Autodesk Inventor part; units mm, degrees
ref_plane "YZ Plane" through (0, 0, 0) normal (1, 0, 0) x (0, 1, 0)
ref_plane "XZ Plane" through (0, 0, 0) normal (0, 1, 0) x (-1, 0, 0)
ref_plane "XY Plane" through (0, 0, 0) normal (0, 0, 1) x (1, 0, 0)
sketch "Boceto1" plane through (0, 0, 0) normal (0, 0, 1) x (1, 0, 0)
  line L0 (250, 0) -> (250, 1160)
  line L1 (0, 1160) -> (0, 0)
  line L2 (230, 20) -> (230, 0)
  line L3 (20, 20) -> (20, 0)
  line L4 (230, 0) -> (230, 140)
  line L5 (230, 140) -> (20, 140)
  line L6 (20, 152.5) -> (230, 152.5)
  line L7 (230, 152.5) -> (230, 457.5)
  line L8 (230, 457.5) -> (20, 457.5)
  line L9 (20, 457.5) -> (20, 470)
  line L10 (20, 470) -> (230, 470)
  line L11 (230, 470) -> (230, 457.5)
  line L12 (230, 470) -> (230, 775)
  line L13 (230, 775) -> (20, 775)
  line L14 (20, 775) -> (20, 787.5)
  line L15 (20, 787.5) -> (230, 787.5)
  line L16 (230, 787.5) -> (230, 775)
  line L17 (230, 787.5) -> (230, 1147.5)
  line L18 (230, 1147.5) -> (20, 1147.5)
  line L19 (20, 1160) -> (230, 1160)
  line L20 (230, 1160) -> (230, 1147.5)
  line L21 (0, 0) -> (20, 0)
  line L22 (230, 0) -> (250, 0)
  line L23 (20, 20) -> (20, 140)
  line L24 (230, 140) -> (230, 20)
  line L25 (20, 152.5) -> (20, 457.5)
  line L26 (230, 1147.5) -> (230, 470)
  line L27 (230, 457.5) -> (230, 152.5)
  line L28 (20, 470) -> (20, 775)
  line L29 (20, 787.5) -> (20, 1147.5)
  line L30 (0, 0) -> (529.2462, 0) construction
  line L31 (20, 1160) -> (0, 1160)
  line L32 (230, 1160) -> (250, 1160)
  line L33 (230, 1147.5) -> (250, 1147.5)
  dimension "d5" = 140
  dimension "d6" = 12.5
  dimension "d7" = 305
  dimension "d8" = 12.5
  dimension "d9" = 305
  dimension "d10" = 12.5
  dimension "d11" = 360
  dimension "d13" = 12.5
  dimension "d28" = 1160
  dimension "d29" = 250
  dimension "d30" = 210
  dimension "d31" = 20
extrude "Extrusión1" add sketch "Boceto1" along normal blind 600 contours L22 L2 L4 L5 L23 L3 L21 L1 L31 L19 L20 L33 L0 | L33 L20 L32 L0 | L16 L13 L14 L15 | L11 L8 L9 L10
sketch "Boceto2" plane through (250, 0, 0) normal (1, 0, 0) x (0, 0, -1)
  line L0 (0, 457.5) -> (0, 152.5)
  line L1 (0, 152.5) -> (0, 457.5)
  line L2 (0, 0) -> (-600, 0)
  line L3 (0, 0) -> (-600, 0)
  line L4 (0, 0) -> (-600, 0)
  line L5 (0, 0) -> (-600, 0)
  line L6 (-600, 140) -> (-600, 0)
  line L7 (0, 140) -> (0, 0)
  line L8 (0, 0) -> (-600, 0)
  line L9 (-600, 140) -> (-600, 0)
  line L10 (0, 140) -> (-600, 140)
  line L11 (0, 0) -> (-600, 0)
  line L12 (0, 0) -> (-600, 0)
  line L13 (0, 140) -> (-600, 140)
  line L14 (0, 0) -> (0, 140)
  line L15 (0, 140) -> (-600, 140)
  line L16 (-600, 0) -> (-600, 140)
  line L17 (0, 0) -> (-600, 0)
  line L18 (0, 140) -> (-600, 140)
  line L19 (0, 140) -> (-600, 140)
  line L20 (0, 152.5) -> (-600, 152.5)
  line L21 (-600, 457.5) -> (-600, 152.5)
  line L22 (0, 457.5) -> (0, 152.5)
  line L23 (0, 152.5) -> (-600, 152.5)
  line L24 (-600, 457.5) -> (-600, 152.5)
  line L25 (0, 457.5) -> (-600, 457.5)
  line L26 (-600, 152.5) -> (-600, 457.5)
  line L27 (0, 152.5) -> (0, 457.5)
  line L28 (0, 457.5) -> (-600, 457.5)
  line L29 (-600, 152.5) -> (-600, 457.5)
  line L30 (0, 152.5) -> (-600, 152.5)
  line L31 (0, 0) -> (0, 1160)
  line L32 (0, 1160) -> (0, 0)
  line L33 (0, 140) -> (0, 0)
  line L34 (0, 0) -> (0, 140)
  line L35 (0, 1160) -> (0, 0)
  line L36 (0, 0) -> (0, 1160)
  line L37 (0, 470) -> (0, 775)
  line L38 (0, 775) -> (0, 470)
  line L39 (0, 152.5) -> (0, 457.5)
  line L40 (0, 457.5) -> (0, 152.5)
  line L41 (-600, 0) -> (-600, 1160)
  line L42 (0, 0) -> (0, 1160)
  line L43 (-600, 0) -> (-600, 1160)
  line L44 (0, 0) -> (-600, 0)
  line L45 (-600, 1160) -> (-600, 0)
  line L46 (0, 1160) -> (0, 0)
  line L47 (0, 0) -> (-600, 0)
  line L48 (-600, 1160) -> (-600, 0)
  line L49 (-600, 140) -> (-600, 0)
  line L50 (-600, 0) -> (-600, 1160)
  line L51 (-600, 1160) -> (-600, 0)
  line L52 (-600, 0) -> (-600, 140)
  line L53 (-600, 470) -> (-600, 775)
  line L54 (-600, 775) -> (-600, 470)
  line L55 (-600, 457.5) -> (-600, 152.5)
  line L56 (-600, 152.5) -> (-600, 457.5)
  line L57 (0, 1600) -> (-600, 1600)
  line L58 (0, 152.5) -> (-600, 152.5)
  line L59 (0, 152.5) -> (-600, 152.5)
  line L60 (0, 152.5) -> (-600, 152.5)
  line L61 (0, 0) -> (-600, 0)
  line L62 (0, 140) -> (-600, 140)
  line L63 (0, 140) -> (0, 0)
  line L64 (-600, 0) -> (-600, 140)
  line L65 (0, 0) -> (-600, 0)
  line L66 (0, 0) -> (0, 140)
  line L67 (0, 1160) -> (-600, 1160)
  line L68 (0, 1160) -> (-600, 1160)
  line L69 (0, 1160) -> (0, 1147.5)
  line L70 (0, 1580) -> (-600, 1580)
  line L71 (0, 1580) -> (-600, 1580)
  line L72 (0, 1580) -> (0, 1160)
  line L73 (-600, 1160) -> (-600, 1147.5)
  line L74 (-600, 470) -> (-600, 775)
  line L75 (0, 457.5) -> (-600, 457.5)
  line L76 (0, 457.5) -> (-600, 457.5)
  line L77 (0, 457.5) -> (-600, 457.5)
  line L78 (0, 457.5) -> (-600, 457.5)
  line L79 (0, 470) -> (-600, 470)
  line L80 (0, 470) -> (-600, 470)
  line L81 (0, 470) -> (-600, 470)
  line L82 (-600, 775) -> (-600, 470)
  line L83 (0, 775) -> (0, 470)
  line L84 (0, 775) -> (0, 470)
  line L85 (0, 470) -> (-600, 470)
  line L86 (-600, 775) -> (-600, 470)
  line L87 (0, 775) -> (-600, 775)
  line L88 (0, 470) -> (0, 775)
  line L89 (0, 470) -> (0, 775)
  line L90 (0, 775) -> (-600, 775)
  line L91 (-600, 470) -> (-600, 775)
  line L92 (0, 470) -> (-600, 470)
  line L93 (0, 470) -> (-600, 470)
  line L94 (0, 775) -> (-600, 775)
  line L95 (0, 775) -> (-600, 775)
  line L96 (0, 775) -> (-600, 775)
  line L97 (0, 775) -> (-600, 775)
  line L98 (0, 787.5) -> (-600, 787.5)
  line L99 (0, 787.5) -> (-600, 787.5)
  line L100 (0, 787.5) -> (-600, 787.5)
  line L101 (0, 787.5) -> (-600, 787.5)
  line L102 (-600, 1147.5) -> (-600, 787.5)
  line L103 (-600, 787.5) -> (-600, 1147.5)
  line L104 (0, 1147.5) -> (-600, 1147.5)
  line L105 (0, 1147.5) -> (0, 787.5)
  line L106 (0, 787.5) -> (-600, 787.5)
  line L107 (-600, 1147.5) -> (-600, 787.5)
  line L108 (0, 1147.5) -> (-600, 1147.5)
  line L109 (0, 787.5) -> (0, 1147.5)
  line L110 (0, 1147.5) -> (-600, 1147.5)
  line L111 (-600, 787.5) -> (-600, 1147.5)
  line L112 (0, 787.5) -> (-600, 787.5)
  line L113 (0, 1147.5) -> (0, 787.5)
  line L114 (0, 787.5) -> (0, 1147.5)
  line L115 (0, 1600) -> (-600, 1600)
  line L116 (0, 1147.5) -> (-600, 1147.5)
  line L117 (0, 1147.5) -> (-600, 1147.5)
  line L118 (0, 1147.5) -> (-600, 1147.5)
  line L119 (0, 1160) -> (-600, 1160)
  line L120 (0, 1160) -> (-600, 1160)
  line L121 (0, 787.5) -> (0, 1147.5)
  line L122 (-600, 787.5) -> (-600, 1147.5)
  line L123 (0, 1580) -> (0, 1160)
  line L124 (0, 1160) -> (-600, 1160)
  line L125 (-600, 1580) -> (-600, 1160)
  line L126 (0, 1580) -> (-600, 1580)
  line L127 (0, 1600) -> (-600, 1600)
  line L128 (0, 1600) -> (-600, 1600)
  line L129 (0, 1580) -> (-600, 1580)
  line L130 (0, 1580) -> (-600, 1580)
  line L131 (-580, 0) -> (-580, 1600)
  line L132 (-20, 1600) -> (-20, 0)
  line L133 (0, 1160) -> (-600, 1160)
  line L134 (0, 1160) -> (-600, 1160)
  line L135 (0, 1147.5) -> (-600, 1147.5)
  line L136 (0, 787.5) -> (-600, 787.5)
  point P0 (-20, 1160)
  point P1 (-20, 1580)
  point P2 (-580, 1580)
  point P3 (-580, 1160)
  point P4 (-20, 787.5)
  point P5 (-20, 1147.5)
  point P6 (-580, 1147.5)
  point P7 (-580, 787.5)
  point P8 (-20, 470)
  point P9 (-20, 775)
  point P10 (-580, 775)
  point P11 (-580, 470)
  point P12 (-20, 152.5)
  point P13 (-20, 457.5)
  point P14 (-580, 457.5)
  point P15 (-580, 152.5)
  point P16 (-20, 140)
  point P17 (-580, 140)
  dimension "d16" = 20
  dimension "d17" = 20
extrude "Extrusión2" cut sketch "Boceto2" against normal blind 600 contours L132 L20 L131 L25 | L79 L131 L87 L132 | L132 L2 L131 L10 | L98 L131 L104 L132
sketch "Boceto3" plane through (250, 0, 0) normal (1, 0, 0) x (0, 0, -1)
  line L0 (-20, 787.5) -> (-580, 787.5)
  line L1 (-20, 1147.5) -> (-580, 1147.5)
  line L2 (-420, 787.5) -> (-180, 787.5)
  line L3 (-180, 1147.5) -> (-420, 1147.5)
  line L4 (-580, 787.5) -> (-580, 1147.5)
  line L5 (-20, 1147.5) -> (-20, 787.5)
  line L6 (-580, 775) -> (-20, 775)
  line L7 (-580, 470) -> (-20, 470)
  line L8 (-420, 775) -> (-180, 775)
  line L9 (-180, 775) -> (-180, 470)
  line L10 (-180, 470) -> (-420, 470)
  line L11 (-420, 470) -> (-420, 775)
  line L12 (-300, 775) -> (-300, 470)
  line L13 (-20, 775) -> (-20, 470)
  point P0 (0, 0)
  dimension "d32" = 240
  dimension "d33" = 160
extrude "Extrusión3" add sketch "Boceto3" against normal blind 10 contours L6 L12 L7 L11 | L6 L9 L7 L12
properties part number "ESTANTERÍA2" material "Aluminio 6061"
Read the model definition and answer for the solid it produces. Units are mm, in the model's axes. A direction names the side the tool comes from. Give positions to 0.01 mm unless a question says otherwise; leave off trailing zeros. Write each loop counter-clockwise with the first axis right and the second up, starting at its lowest first coordinate (ties: lowest second). Pieces come first, ordered by that corner, then holes. Notation, with made-up numbers: M 81,82 L 126,82 A23 cw 126,115 Z; hole C -0.75,1.5 d5. An arc over 180 degrees is marked long. One line per item, written item: value. Start each with the question number.
(1) Find section B-B (z = 245.5). Determine the outline of the cut face in (x, y).
(2) Find section A-A (x = 111). Determine the outline of the cut face in (y, z), plus the area to 3 significant figures.
(3) Find section D-D (z = 167.5). Determine the outline of the cut face in (x, y), plus the area to 3 significant figures.
(4) A flat-ended cylindrical pin translates along its axis: pin 1 Ø8 at (x, z) = (45, 124.5) entering from -Y. Find the tip coordinate at first contact, or state that the pin passes through.
(5) A tool of negligible diameter and unlimited length cuts with its end or side. For faces 1 (the flat face through (230, 71, 590)), 2 (the flat face through (20, 303, 10)), 3 (the flat face through (240, 303, 580)), from which of +Z, -Z, +X, -X, +Y, -Y can it reach the whole face along a straight path? Write none if from no direction.
(6) Find the intervals of material crossed by line 1 (Y direction, x = 62, z = 113.5); line 2 (Z direction, x = 17.5, y = 979), in increasing order.
(7) Determine the mould class of faces 4 (the flat face through (230, 620, 590)), 5 (the flat face through (240, 970, 20)), 6 (the flat face through (13, 583, 600)) for opening direction Z: pulls with the +Z half, pulls with the -Z half, needs draft (parallel to the pull), parting line crosses it, or undercut.
(8) Find section C-C (y = 545.5). Determine the outline of the cut face in (x, z).
Results below:
1. outline: M 0,140 L 250,140 L 250,152.5 L 0,152.5 Z; M 0,457.5 L 250,457.5 L 250,787.5 L 0,787.5 L 0,775 L 240,775 L 240,470 L 0,470 Z; M 0,1147.5 L 250,1147.5 L 250,1160 L 0,1160 Z
2. outline: M 140,0 L 152.5,0 L 152.5,600 L 140,600 Z; M 457.5,0 L 470,0 L 470,600 L 457.5,600 Z; M 775,0 L 787.5,0 L 787.5,600 L 775,600 Z; M 1147.5,0 L 1160,0 L 1160,600 L 1147.5,600 Z
2. area: 30,000 mm^2
3. outline: M 0,140 L 250,140 L 250,152.5 L 0,152.5 Z; M 0,457.5 L 250,457.5 L 250,470 L 0,470 Z; M 0,775 L 250,775 L 250,787.5 L 0,787.5 Z; M 0,1147.5 L 250,1147.5 L 250,1160 L 0,1160 Z
3. area: 12,500 mm^2
4. pin 1: stops at y = 140
5. face 1: +Z, -Z, -Y
5. face 2: +Z, -Z
5. face 3: +X, -X
6. line 1: y = 140 to 152.5, 457.5 to 470, 775 to 787.5, 1147.5 to 1160
6. line 2: z = 0 to 20, 580 to 600
7. face 4: needs draft
7. face 5: undercut
7. face 6: pulls with the +Z half
8. outline: M 0,0 L 20,0 L 20,20 L 0,20 Z; M 0,580 L 20,580 L 20,600 L 0,600 Z; M 230,0 L 250,0 L 250,20 L 230,20 Z; M 230,580 L 250,580 L 250,600 L 230,600 Z; M 240,180 L 250,180 L 250,420 L 240,420 Z
